Part model, mm, in its own coordinate system. Face numbers are marked on the shaded views. A direction names the side the tool comes from. Round coordinates to 2 decimals unless told otherwise and drop trailing zeros. Loops run counter-clockwise (first coordinate to the right, second up) from the corner with the lowest first, then second, coordinate; pieces in that order, holes last. Notation, with made-up numbers: (13, 14) -> (59, 14) arc R34 ccw to (59, 45) -> close; hole circle Ø6 at (67, 50). An arc over 180 degrees is marked (long way). Answer as CSV lines item,"result".
from build123d import *

# Parameters (mm, degrees)
F0_W     = 13
F0_H     = 13
F0_R     = 3
F0_R_2   = 1.25
F1_DEPTH = 3
F2_DEPTH = 7
F3_DEPTH = 10
F4_R     = 2


with BuildPart() as f1:
    # F0 (on Top) → F1 (new body)
    with BuildSketch(Plane.XY):
        with Locations((6.5, 6.5)):
            Rectangle(F0_W, F0_H)
        with Locations((6.5, 6.5)):
            Circle(F0_R, mode=Mode.SUBTRACT)
        with Locations((6.5, 6.5)):
            Circle(F0_R)
        with Locations((6.5, 6.5)):
            Circle(F0_R_2, mode=Mode.SUBTRACT)
        with Locations((6.5, 6.5)):
            Circle(F0_R_2)
    extrude(amount=F1_DEPTH)

    # F0 (on Top) → F2 (join)
    with BuildSketch(Plane.XY):
        with Locations((6.5, 6.5)):
            Circle(F0_R)
        with Locations((6.5, 6.5)):
            Circle(F0_R_2, mode=Mode.SUBTRACT)
        with Locations((6.5, 6.5)):
            Circle(F0_R_2)
    extrude(amount=F2_DEPTH)

    # F0 (on Top) → F3 (join)
    with BuildSketch(Plane.XY):
        with Locations((6.5, 6.5)):
            Circle(F0_R_2)
    extrude(amount=F3_DEPTH)

    # F4
    f4_edges = [f1.edges().sort_by_distance(p)[0] for p in [
        (3.5, 6.5, 3),
    ]]
    fillet(f4_edges, radius=F4_R)


solid = f1.part
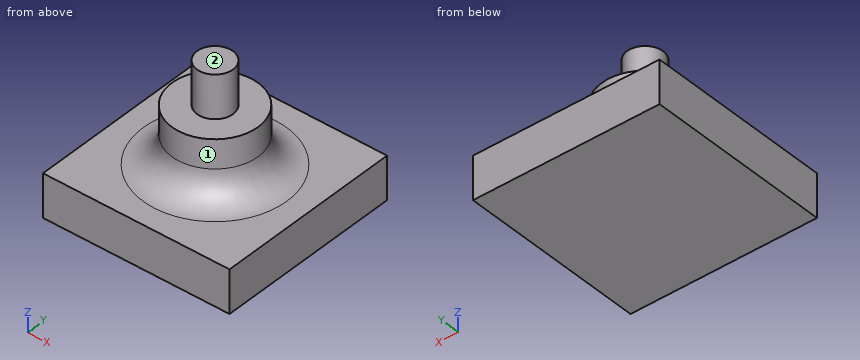
Q1. Saw through at D-D, the plane y = 1. Write the cut outline in (x, z), then the cut area to 3 significant figures.
Geometry results:
outline,"(0, 0) -> (13, 0) -> (13, 3) -> (0, 3) -> close"
area,"39.0 mm2"
Q2. Saw through at A-A, the plane y = 6.5. Write the cut outline in (x, z), then the cut area to 3 significant figures.
Geometry results:
outline,"(0, 0) -> (13, 0) -> (13, 3) -> (11.5, 3) arc R2 cw to (9.5, 5) -> (9.5, 7) -> (7.75, 7) -> (7.75, 10) -> (5.25, 10) -> (5.25, 7) -> (3.5, 7) -> (3.5, 5) arc R2 cw to (1.5, 3) -> (0, 3) -> close"
area,"72.2 mm2"
Q3. Saw through at C-C, the plane z = 6.25. Write the cut outline in (x, y), then the cut area to 3 significant figures.
Geometry results:
outline,"circle Ø6 at (6.5, 6.5)"
area,"28.3 mm2"
Q4. Drop flat-ended pins along their axis: P1, Ø1, axis at x = 5, z = 4.5, coming from the +Y side; P2, Ø1, axis at x = 9, z = 5.5, coming from the +Y side; P3, Ø4, axis at x = 1.5, y = 9, coming from the +Z side; P4, Ø1.5, axis at x = 4.5, y = 6, coming from the -Z side. Give the stop position or say it passes through.
Geometry results:
P1,"y = 9.48"
P2,"y = 8.74"
P3,"z = 3.58"
P4,"z = 0"
Q5. Drill centre lines: line 1 along Z through (x, y) = (1, 1); line 2 along Z through (x, y) = (8.25, 6); line 3 along X through (y, z) = (6.5, 5). Where is each one in solid material? Low to high.
Geometry results:
line 1,"0 to 3"
line 2,"0 to 7"
line 3,"3.5 to 9.5"
Q6. Which spindle directions (+Z, -Z, +X, -X, +Y, -Y) get a long thin tool onto all of the face, cutting with end or side? Do the marked faces 1 and 2. Say none if no direction does.
Geometry results:
face 1,"+Z"
face 2,"+Z, +X, -X, +Y, -Y"
